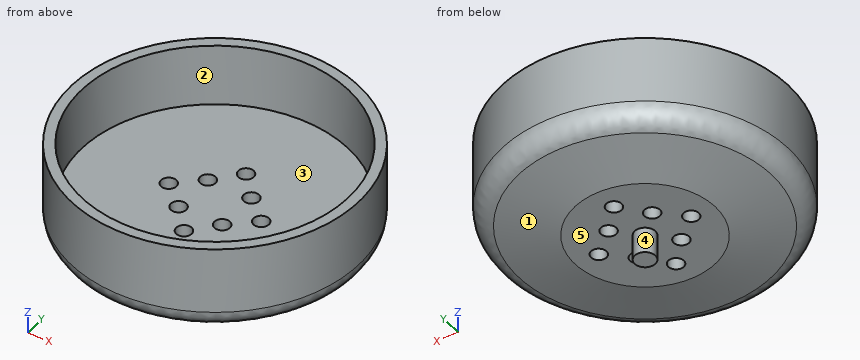
from build123d import *

# Parameters (mm, degrees)
SKETCH3_R          = 1.5
CUT_EXTRUDE1_DEPTH = 19.75
CIRPATTERN1_COUNT  = 4
CHAMFER1_SIZE      = 2.5
CHAMFER1_SIZE2     = 14.178204549
FILLET1_R          = 4
SKETCH4_R          = 25.8
CUT_EXTRUDE2_DEPTH = 12


with BuildPart() as part:
    # Sketch2 → Revolve1 (revolve)
    with BuildSketch(Plane(origin=(0, 0, 0), x_dir=(1, 0, 0), z_dir=(0, 1, 0))):
        Polygon((0, 32), (-2, 32), (-2, 27), (-27.8, 27), (-27.8, 8.25), (0, 8.25), align=None)
    revolve(axis=Axis((0, 0, -88.99), (0, 0, 1)))

    # Sketch3 → Cut-Extrude1 (cut, through all)
    with BuildSketch(Plane(origin=(0, 0, -27), x_dir=(-1, 0, 0), z_dir=(0, 0, -1))):
        with Locations((0, 9)):
            Circle(SKETCH3_R)
        with Locations((4.242640687, 4.242640687)):
            Circle(SKETCH3_R)
    cut_extrude1 = extrude(amount=-CUT_EXTRUDE1_DEPTH, mode=Mode.SUBTRACT)

    # CirPattern1: Cut-Extrude1 ×4 about axis
    cirpattern1_axis = Axis((0, 0, 0), (0, 0, 1))
    for i in range(1, CIRPATTERN1_COUNT):
        add(cut_extrude1.rotate(cirpattern1_axis, i * 360 / CIRPATTERN1_COUNT), mode=Mode.SUBTRACT)

    # Chamfer1
    chamfer1_edges = [part.edges().sort_by_distance(p)[0] for p in [
        (27.8, 0, -27),
    ]]
    chamfer1_side = [part.faces().sort_by_distance(p)[0] for p in [
        (27.8, 0, -17.625),
    ]]
    chamfer(chamfer1_edges, length=CHAMFER1_SIZE, length2=CHAMFER1_SIZE2, reference=chamfer1_side[0])

    # Fillet1
    fillet1_edges = [part.edges().sort_by_distance(p)[0] for p in [
        (27.8, 0, -24.5),
    ]]
    fillet(fillet1_edges, radius=FILLET1_R)

    # Sketch4 → Cut-Extrude2 (cut)
    with BuildSketch(Plane.XY.offset(-8.25)):
        Circle(SKETCH4_R)
    extrude(amount=-CUT_EXTRUDE2_DEPTH, mode=Mode.SUBTRACT)


solid = part.part
CAD build for the part. Positions are in the model's coordinates, mm. Face numbers are marked on the shaded views. A direction names the side the tool comes from. Round coordinates to 2 decimals unless told otherwise and drop trailing zeros. Write each loop counter-clockwise with the first axis right and the second up, starting at its lowest first coordinate (ties: lowest second). Pieces come first, ordered by that corner, then holes. Notation, with made-up numbers: M -25,29.25 L 21,29.25 A30 ccw 21,54.25 Z; hole C 77.5,80 d11. An arc over 180 degrees is marked long. Put each result on its own line as item: value. Start each with the question number.
1) Pin check, flat tips, straight feed: pin 1 Ø2 at (x, y) = (4.5, 2.5) entering from -Z; pin 2 Ø5 at (x, y) = (4.24, -4.24) entering from +Z; pin 3 Ø2.5 at (x, y) = (-9, 0) entering from +Z; pin 4 Ø10 at (x, z) = (-9.5, -11) entering from +Y. Stop position of each tip, or through.
2) Drill centre lines: probe 1 along X at (y, z) = (0, -24.5); probe 2 along X at (y, z) = (0, -23); probe 3 along Y at (x, z) = (8.5, -18.5). Where is each one in solid material? Low to high. Write a range as [from, to].
3) 3-axis set-ups, long thin cutter, end or side, ignore diameter. For the marked faces 1 and 2: which of +Z, -Z, +X, -X, +Y, -Y reach the whole face in a straight line?
4) Saw through at A-A, the plane z = -16.25. Write the cut outline in (x, y).
5) Saw through at B-B, the plane x = 0. Count the separate pieces of the cut face and the enclosed holes in it, and give its area (3 significant figures).
6) Pull direction X, two halves, no side cores. Call the marked faces 3, 4 and 5: pulls with the +X half, pulls with the -X half, needs draft (parallel to the pull), parting line crosses it, or undercut.
Resolved:
1. pin 1: z = -27
1. pin 2: z = -20.25
1. pin 3: through
1. pin 4: y = 27.43
2. probe 1: [-25.98, -10.5], [-7.5, 7.5], [10.5, 25.98]
2. probe 2: [-27.34, -10.5], [-7.5, 7.5], [10.5, 27.34]
2. probe 3: [-26.47, -24.36], [24.36, 26.47]
3. face 1: -Z
3. face 2: +Z
4. outline: C 0,0 d55.6; hole C 0,0 d51.6
5. separate pieces: 3
5. enclosed holes: 0
5. area: 363 mm²
6. face 3: undercut
6. face 4: parting line crosses it
6. face 5: needs draft
